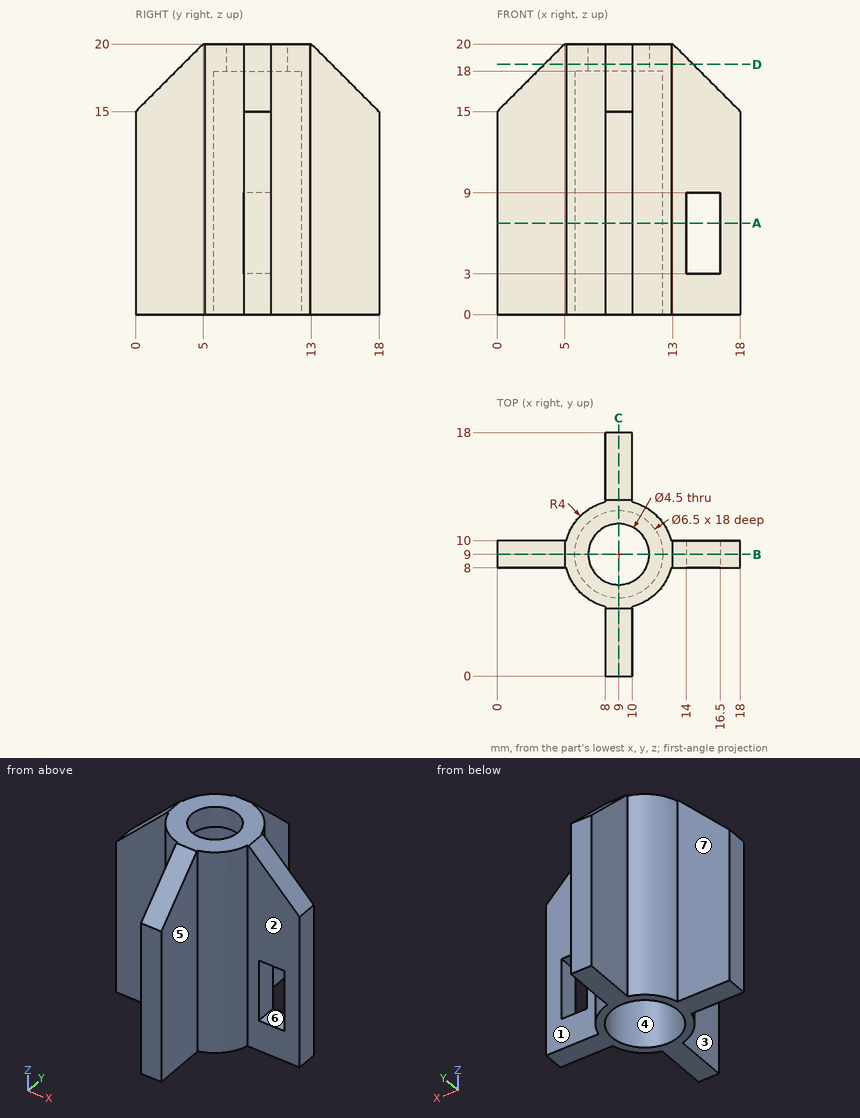
Job drawing, mm, ordinate dimensions from the low corner. One solid piece. A direction names the side the tool comes from. Give positions to 0.01 mm unless a question says otherwise; leave off trailing zeros. Order: outer loops, then holes, each group sorted by start corner. A loop starts at its lowest first (then second) coordinate and runs counter-clockwise, first axis right, second up. Notation, with made-up numbers: M 33,47 L 49,47 A20 ccw 49,70 Z; hole C -15.5,23.25 d3. An arc over 180 degrees is marked long. Return JSON: item names as keys, results as strings.
Q1. Two-plate mould, pull along X, no slides. Class the marked faces 4, 5, 6 and 7: pulls with the +X half, pulls with the -X half, needs draft (parallel to the pull), parting line crosses it, or undercut.
Answer list:
{"face 4": "undercut", "face 5": "pulls with the +X half", "face 6": "undercut", "face 7": "needs draft"}
Q2. Band-saw the part on C-C (x = 9). Give the cut face in (y, z).
Answer list:
{"outline": "M 0,0 L 5.75,0 L 5.75,18 L 6.75,18 L 6.75,20 L 5,20 L 0,15 Z; M 11.25,18 L 12.25,18 L 12.25,0 L 18,0 L 18,15 L 13,20 L 11.25,20 Z"}
Q3. Band-saw the part on D-D (z = 18.5). Give the cut face in (x, y), then the cut area to 3 significant figures.
Answer list:
{"outline": "M 3.5,8 L 5.13,8 A4 ccw 8,5.13 L 8,3.5 L 10,3.5 L 10,5.13 A4 ccw 12.87,8 L 14.5,8 L 14.5,10 L 12.87,10 A4 ccw 10,12.87 L 10,14.5 L 8,14.5 L 8,12.87 A4 ccw 5.13,10 L 3.5,10 Z; hole C 9,9 d4.5", "area": "46.7 mm^2"}
Q4. Flat gauge pins, fed straight in: pin 1 (3 mm diameter, centred on y = 5, z = 13, fed in from -X); pin 2 (5.5 mm diameter, centred on x = 1.5, z = 8, fed in from -Y); pin 3 (3 mm diameter, centred on x = 8, y = 9, fed in from -Z). Where does each tip first touch, or does it go through?
Answer list:
{"pin 1": "stops at x = 5.88", "pin 2": "stops at y = 8", "pin 3": "stops at z = 18"}
Q5. Band-saw the part on A-A (z = 6.75). Give the cut face in (x, y).
Answer list:
{"outline": "M 0,8 L 5.13,8 A4 ccw 8,5.13 L 8,0 L 10,0 L 10,5.13 A4 ccw 12.87,8 L 14,8 L 14,10 L 12.87,10 A4 ccw 10,12.87 L 10,18 L 8,18 L 8,12.87 A4 ccw 5.13,10 L 0,10 Z; M 16.5,8 L 18,8 L 18,10 L 16.5,10 Z; hole C 9,9 d6.5"}
Q6. Wall check: probe 1 along Y at (x, z) = (9, 7.5); probe 2 along Y at (x, z) = (7.25, 14.5); probe 3 along Y at (x, z) = (1, 3.75). Give the ranges that are in metal, low to high. Write a range as from..to.
Answer list:
{"probe 1": "y = 0..5.75, 12.25..18", "probe 2": "y = 5.4..6.26, 11.74..12.6", "probe 3": "y = 8..10"}
Q7. Band-saw the part on B-B (y = 9). Give the cut face in (x, z).
Answer list:
{"outline": "M 0,0 L 5.75,0 L 5.75,18 L 6.75,18 L 6.75,20 L 5,20 L 0,15 Z; M 11.25,18 L 12.25,18 L 12.25,0 L 18,0 L 18,15 L 13,20 L 11.25,20 Z; hole M 14,3 L 16.5,3 L 16.5,9 L 14,9 Z"}
Q8. 3-axis set-ups, long thin cutter, end or side, ignore diameter. For the marked faces 1, 2 and 3: which of +Z, -Z, +X, -X, +Y, -Y reach the whole face in a straight line?
Answer list:
{"face 1": "+Z, -Z, +X, +Y", "face 2": "+Z, -Z, +X, -Y", "face 3": "+Z, -Z, -X, -Y"}
